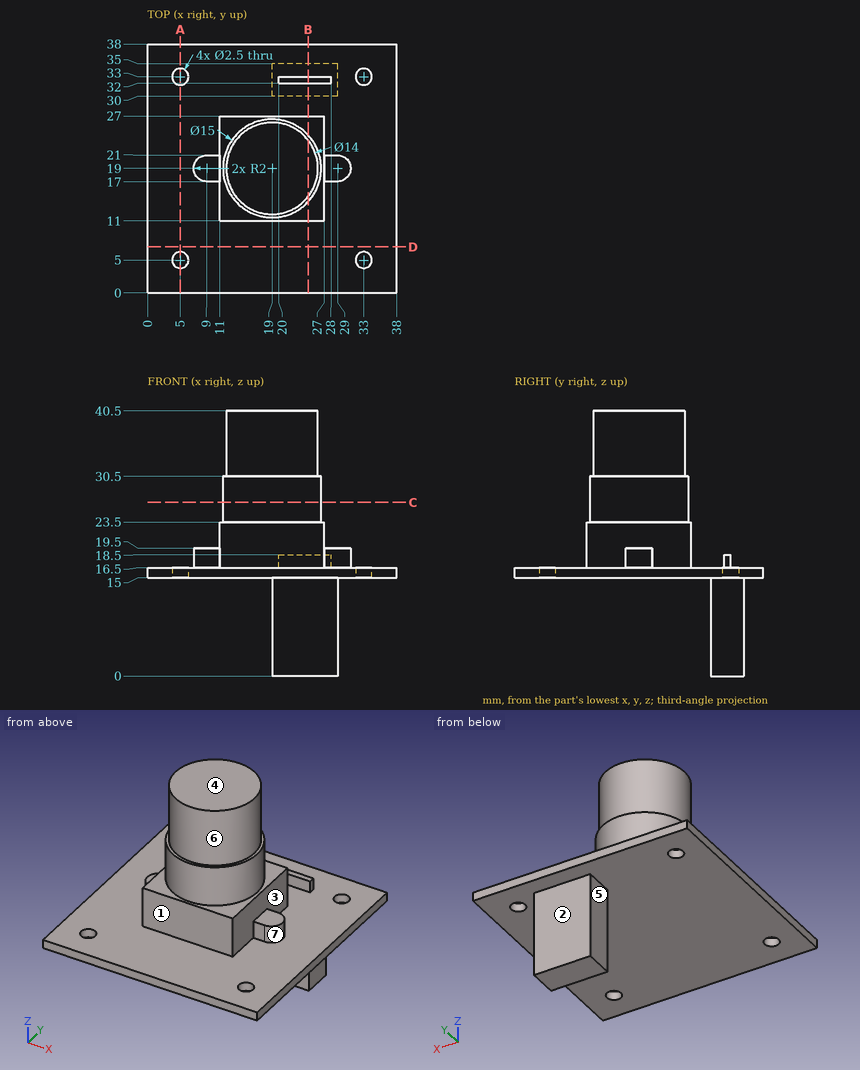
Source: three-view drawing plus pictorial views. Frame: mm from the lowest corner of the part. A direction names the side the tool comes from. Give positions to 0.01 mm unless a question says otherwise; leave off trailing zeros. Write each loop counter-clockwise with the first axis right and the second up, starting at its lowest first coordinate (ties: lowest second). Pieces come first, ordered by that corner, then holes. Notation, with made-up numbers: (-9.75, -27) - (45.25, -27) arc R7 cw to (45.25, -19) - close; hole circle Ø7 at (-17.5, 8.5). An arc over 180 degrees is marked (long way). Write item = value, one per line. Start each with the question number.
Q1. Reachability of the marked faces 5, 6 and 7 from +Z, -Z, +X, -X, +Y, -Y: full face, straight path, thin tool, end or side. Return the list, or none.
Q2. Cut plane A-A, the plane x = 5. Return loops of the section in (y, z), then the cut area to 3 significant figures.
Q3. Cut plane C-C, the plane z = 26.5. Return loops of the section in (x, y).
Q4. Cut plane D-D, the plane y = 7. Return loops of the section in (x, z).
Q5. Material intervals for probe 1 along X at (y, z) = (33, 15.55); probe 2 along Z at (x, y) = (29, 26), sorted ascending.
Q6. Draft query along Y for the marked faces 1, 2, 3 and 4. Return one class per face: +Y half, -Y half, draft (parallel to the pull), parting line (faces both ways), or undercut.
Q7. Cut plane B-B, the plane x = 24.5. Return loops of the section in (y, z).
Q8. Pin query (flat end, axial travel): pin 1 Ø12 at (y, z) = (23.5, 35.5) entering from -X; pin 2 Ø2 at (x, y) = (5, 33) entering from +Z (3 decimals); pin 3 Ø1.5 at (x, y) = (34, 14.5) entering from +Z; pin 4 Ø0.5 at (y, z) = (32.5, 17.5) entering from -X. Return the tip coordinate at first contact, or that it passes through.
Computed values:
q1.face_5 = -Z, -X, +Y, -Y
q1.face_6 = +Z
q1.face_7 = +Z, +X
q2.outline = (0, 15) - (3.75, 15) - (3.75, 16.5) - (0, 16.5) - close; (6.25, 15) - (31.75, 15) - (31.75, 16.5) - (6.25, 16.5) - close; (34.25, 15) - (38, 15) - (38, 16.5) - (34.25, 16.5) - close
q2.area = 49.5 mm²
q3.outline = circle Ø15 at (19, 19)
q4.outline = (0, 15) - (38, 15) - (38, 16.5) - (0, 16.5) - close
q5.probe_1 = 0 to 3.75, 6.25 to 31.75, 34.25 to 38
q5.probe_2 = 15 to 16.5
q6.face_1 = -Y half
q6.face_2 = +Y half
q6.face_3 = undercut
q6.face_4 = draft
q7.outline = (0, 15) - (30, 15) - (30, 0) - (35, 0) - (35, 15) - (38, 15) - (38, 16.5) - (33, 16.5) - (33, 18.5) - (32, 18.5) - (32, 16.5) - (27, 16.5) - (27, 23.5) - (24.1, 23.5) - (24.1, 30.5) - (23.33, 30.5) - (23.33, 40.5) - (14.67, 40.5) - (14.67, 30.5) - (13.9, 30.5) - (13.9, 23.5) - (11, 23.5) - (11, 16.5) - (0, 16.5) - close
q8.pin_1 = 11.59
q8.pin_2 = through
q8.pin_3 = 16.5
q8.pin_4 = 20
